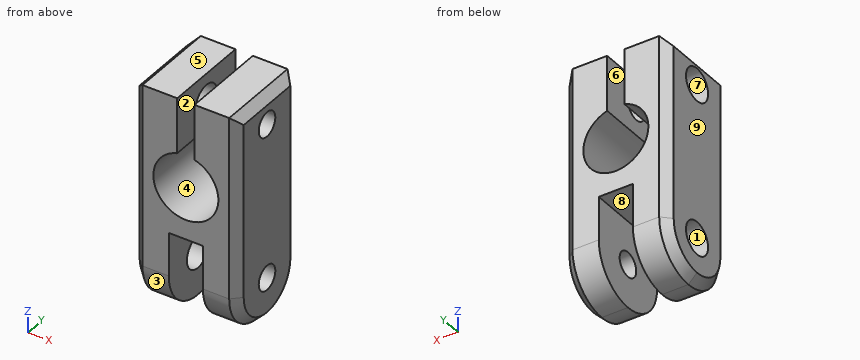
Autodesk Inventor part; units mm, degrees
ref_plane "YZ Plane" through (0, 0, 0) normal (1, 0, 0) x (0, 1, 0)
ref_plane "XZ Plane" through (0, 0, 0) normal (0, 1, 0) x (-1, 0, 0)
ref_plane "XY Plane" through (0, 0, 0) normal (0, 0, 1) x (1, 0, 0)
sketch "Sketch1" plane through (0, 0, 0) normal (0, 1, 0) x (-1, 0, 0)
  circle A0 centre (0, 0) radius 4.7625
  line L0 (7.62, -20.32) -> (-7.62, -20.32)
  line L1 (-7.62, -20.32) -> (-7.62, 12.7)
  line L2 (-7.62, 12.7) -> (7.62, 12.7)
  line L3 (7.62, 12.7) -> (7.62, -20.32)
  line L4 (1.27, 4.59) -> (1.27, 12.7)
  line L5 (-1.27, 4.59) -> (-1.27, 12.7)
  line L6 (0, 4.7625) -> (0, 12.7) construction
  dimension "d0" = 9.525
  dimension "d1" = 7.62
  dimension "d2" = 7.62
  dimension "d3" = 20.32
  dimension "d4" = 12.7
  dimension "d6" = 1.27
  dimension "d7" = 1.27
extrude "Extrusion1" add sketch "Sketch1" along normal blind 12.7 contours A0 L4 L2 L3 L0 L1 L5
sketch "Sketch2" plane through (-7.62, 0, -20.32) normal (-1, 0, 0) x (0, 0, 1)
  line L0 (0, 0) -> (33.02, 0)
  line L1 (33.02, 0) -> (33.02, 12.7)
  line L2 (0, 12.7) -> (33.02, 12.7)
  line L3 (0, 0) -> (0, 12.7)
  line L4 (0, 6.35) -> (33.02, 6.35) construction
  circle A0 centre (28.9687, 6.35) radius 1.75
  circle A1 centre (6.35, 6.35) radius 1.5
  point P0 (20.32, 0)
  dimension "d10" = 3.5
  dimension "d11" = 4.0513
  dimension "d20" = 3
  dimension "d21" = 6.35
hole "Hole1" at (-7.62, 6.35, 8.6487) at (-7.62, 6.35, -13.97) direction (1, 0, 0) diameter 3.6068 end through all
fillet "Fillet1" radius 6.35 2 edges at (0, 12.7, -20.32) (0, 0, -20.32)
sketch "Sketch3" plane through (0, 12.7, 0) normal (0, 1, 0) x (1, 0, 0)
  line L0 (-7.62, 13.97) -> (7.62, 13.97)
  line L1 (-7.62, 13.97) -> (-7.62, -12.7)
  line L2 (-7.62, -12.7) -> (-1.27, -12.7)
  line L3 (-1.27, -12.7) -> (-1.27, -4.59)
  arc A0 (1.27, -4.59) -> (-1.27, -4.59) centre (0, 0) ccw
  line L4 (1.27, -4.59) -> (1.27, -12.7)
  line L5 (1.27, -12.7) -> (7.62, -12.7)
  line L6 (7.62, -12.7) -> (7.62, 13.97)
  line L7 (0, 4.7625) -> (0, 20.32) construction
  line L8 (7.62, 20.32) -> (-7.62, 20.32)
  line L9 (2.5, 4.0536) -> (2.5, 20.32)
  line L10 (-2.5, 4.0536) -> (-2.5, 20.32)
  line L11 (2.5, 7.62) -> (-2.5, 7.62)
  dimension "d22" = 2.5
  dimension "d23" = 2.5
  dimension "d26" = 12.7
extrude "Extrusion2" cut sketch "Sketch3" against normal through all contours L10 L8 L9 L0 | L0 L9 L11 L10
chamfer "Chamfer1" distance 1.27 angle 45 8 edges at (-7.62, 0, -0.6352) (-7.62, 10.8403, -18.4603) (-7.62, 12.7, -0.6352) (7.62, 12.7, -0.6353) (7.62, 10.8403, -18.4603) (7.62, 0, -0.6353) (-7.62, 6.35, 12.7) (7.62, 6.35, 12.7)
hole "Hole2" at (-7.62, 6.35, -13.97) at (-7.62, 6.35, 8.6487) direction (1, 0, 0) diameter 4.8006 depth 6.35
equation "\"d2\" = d1"
equation "\"d7\" = d6"
equation "\"d23\" = d22"
Part model, mm, in its own coordinate system. Face numbers are marked on the shaded views. A direction names the side the tool comes from. Give positions to 0.01 mm unless a question says otherwise; leave off trailing zeros. Loops run counter-clockwise (first coordinate to the right, second up) from the corner with the lowest first, then second, coordinate; pieces in that order, holes last. Notation, with made-up numbers: (86, -4.75) -> (144, -4.75) arc R12 ccw to (144, -0.75) -> close; hole circle Ø9 at (-20.5, 52). An arc over 180 degrees is marked (long way). Write each question's results on one line, items separated by ' | '. Start each with the question number.
Q1. Pull direction Z, two halves, no side cores. Call the marked faces 1, 2, 3 and 4: +Z half, -Z half, draft (parallel to the pull), parting line (faces both ways), or undercut.
Q2. Which spindle directions (+Z, -Z, +X, -X, +Y, -Y) get a long thin tool onto all of the face, cutting with end or side? Do the marked faces 5, 6, 7, 8 and 9. Say none if no direction does.
Q3. Band-saw the part on A-A on x = 4. Count the separate pieces of the cut face and the enclosed holes in it, plus the area to 3 significant figures.
Q4. Wall check: L1, parallel to Z at x = 5.5, y = 6.35; L2, parallel to X at y = 8.75, z = -12.5; L3, parallel to Y at x = -6.35, z = -13.97. Give the ranges that are in metal, low to high.
Q5. Pin check, flat tips, straight feed: P1, Ø4, axis at x = -1, y = 4, coming from the -Z side; P2, Ø1.5, axis at x = 0.5, y = 7.5, coming from the -Z side. Stop position of each tip, or through.
Q6. Band-saw the part on D-D on z = -5.5. List the corners of the cut face in (x, y).
Q7. Band-saw the part on B-B on z = 5. List the corners of the cut face in (x, y), plus the area to 3 significant figures.
Results are:
1) face 1: undercut | face 2: draft | face 3: -Z half | face 4: undercut
2) face 5: +Z, +X, -X, +Y, -Y | face 6: +Z, +Y, -Y | face 7: -X | face 8: -Z, +Y, -Y | face 9: +Z, -Z, -X, +Y, -Y
3) separate pieces: 2 | enclosed holes: 2 | area: 316 mm²
4) L1: z = -20.32 to -15.77, -12.17 to 6.85, 10.45 to 12.7 | L2: x = -7.62 to -2.5, 2.5 to 7.62 | L3: y = 0 to 3.95, 8.75 to 12.7
5) P1: stops at z = -20.24 | P2: stops at z = -7.62
6) outline: (-7.62, 1.27) -> (-6.35, 0) -> (6.35, 0) -> (7.62, 1.27) -> (7.62, 11.43) -> (6.35, 12.7) -> (-6.35, 12.7) -> (-7.62, 11.43) -> close
7) outline: (-7.62, 1.27) -> (-6.35, 0) -> (-1.27, 0) -> (-1.27, 12.7) -> (-6.35, 12.7) -> (-7.62, 11.43) -> close; (1.27, 0) -> (6.35, 0) -> (7.62, 1.27) -> (7.62, 11.43) -> (6.35, 12.7) -> (1.27, 12.7) -> close | area: 158 mm²
